Could you check a few things on this model? Use its own coordinates, in mm. Face numbers are marked on the shaded views. A direction names the side the tool comes from. Give positions to 0.01 mm unless a question says otherwise; leave off trailing zeros. Loops run counter-clockwise (first coordinate to the right, second up) from the corner with the lowest first, then second, coordinate; pieces in that order, holes last. Notation, with made-up numbers: (40, 22) - (84, 22) arc R22 cw to (84, 51) - close; hole circle Ø10 at (-3.5, -26.5). An arc over 180 degrees is marked (long way). One line per item, written item: value. Start each with the question number.
Q1. If I drill on line 1 (Y direction, x = -58, z = -8.25); line 2 (X direction, y = -24, z = -9.5); line 3 (X direction, y = 20.5, z = 1.25), over which ranges is the centre line in solid material (lowest first)? Write a range as from..to.
Q2. I'm going to push flat-ended pins straight in: P1, Ø13, axis at x = 17, y = -5, coming from the -Z side; P2, Ø2, axis at x = 47.5, y = 25, coming from the +Z side. Where does each tip first touch, or does it pass through?
Q3. I want a section at C-C (x = -19). Please give me the cut outline in (y, z).
Q4. I want a section at A-A (x = 0). Please give me the cut outline in (y, z), then the cut area to 3 significant figures.
Q5. I want a section at B-B (z = -1.75). Please give me the cut outline in (x, y), then the cut area to 3 significant figures.
Q6. For the marked faces 1, 2 and 3, which set-ups out of +Z, -Z, +X, -X, +Y, -Y let a thin tool reach every point of the face, with its end or its side?
Q7. If we mould it in two halves opening along Y, with no side actions, what happens to the marked faces 4, 5 and 6? For each: released by +Y, released by -Y, zero draft, split by the parting line, or undercut.
```python
from build123d import *

# Parameters (mm, degrees)
F0_W     = 126
F0_H     = 66
F0_W_2   = 120
F0_H_2   = 60
F1_DEPTH = 21
F2_W     = 126
F2_H     = 66
F3_DEPTH = 1
F0_R     = 12
F4_DEPTH = 8
F6_DEPTH = 22


with BuildPart() as f1:
    # F0 (on Top) → F1 (new body)
    with BuildSketch(Plane.XY):
        with Locations((-1.5, -1.5)):
            Rectangle(F0_W, F0_H)
        with Locations((-1.5, -1.5)):
            Rectangle(F0_W_2, F0_H_2, mode=Mode.SUBTRACT)
    extrude(amount=-F1_DEPTH)

    # F2 (on face) → F3 (join)
    with BuildSketch(Plane.XY):
        with Locations((-1.5, -1.5)):
            Rectangle(F2_W, F2_H)
    extrude(amount=F3_DEPTH)

    # F0 (on Top) → F4 (join)
    with BuildSketch(Plane.XY):
        with Locations((-40.3844975889, 14.0422494113)):
            Circle(F0_R)
        with Locations((0, 14)):
            Circle(F0_R)
        with Locations((-40.3844975889, -15.6422494113)):
            Circle(F0_R)
        with Locations((0, -15.6)):
            Circle(F0_R)
        with Locations((40.3844975889, -15.6422494113)):
            Circle(F0_R)
        with Locations((40.3844975889, 14.0422494113)):
            Circle(F0_R)
    extrude(amount=F4_DEPTH)

    # F5 (on face) → F6 (join)
    with BuildSketch(Plane.XY):
        with BuildLine():
            ThreePointArc((31.4784805761, 5.99968384), (32.8922690999, 2.7143222033), (33.3752768321, -0.8295602165))
            ThreePointArc((33.3752768321, -0.8295602165), (32.9180007232, -4.2794585958), (31.5777529034, -7.4910993057))
            ThreePointArc((31.5777529034, -7.4910993057), (33.0771463209, -6.123708691), (34.7855065256, -5.0285177832))
            ThreePointArc((34.7855065256, -5.0285177832), (35.2271141548, -2.9496471052), (35.3752768321, -0.8295602165))
            ThreePointArc((35.3752768321, -0.8295602165), (35.2220188743, 1.3264920966), (34.7653269231, 3.4391875409))
            ThreePointArc((34.7653269231, 3.4391875409), (33.0099261031, 4.57569273), (31.4784805761, 5.99968384))
        make_face()
        with BuildLine():
            ThreePointArc((30.044931449, 7.9518165828), (30.8064288175, 7.0085924135), (31.4784805761, 5.99968384))
            ThreePointArc((31.4784805761, 5.99968384), (33.0099261031, 4.57569273), (34.7653269231, 3.4391875409))
            ThreePointArc((34.7653269231, 3.4391875409), (32.4184567267, 8.1923854782), (28.5856333111, 11.8543733283))
            ThreePointArc((28.5856333111, 11.8543733283), (29.1446126861, 9.8392757768), (30.044931449, 7.9518165828))
        make_face()
        with BuildLine():
            ThreePointArc((34.7855065256, -5.0285177832), (33.0771463209, -6.123708691), (31.5777529034, -7.4910993057))
            ThreePointArc((31.5777529034, -7.4910993057), (30.8212956484, -8.6474276201), (29.948463719, -9.718635897))
            ThreePointArc((29.948463719, -9.718635897), (29.0995516946, -11.5618087289), (28.5733528944, -13.5216690648))
            ThreePointArc((28.5733528944, -13.5216690648), (32.4355688891, -9.8281570151), (34.7855065256, -5.0285177832))
        make_face()
        with BuildLine():
            ThreePointArc((10.5845976874, 8.3461259481), (20.4011056558, 12.410159384), (30.044931449, 7.9518165828))
            ThreePointArc((30.044931449, 7.9518165828), (29.1446126861, 9.8392757768), (28.5856333111, 11.8543733283))
            ThreePointArc((28.5856333111, 11.8543733283), (20.2186418923, 14.4126354365), (11.8233794228, 11.9487323369))
            ThreePointArc((11.8233794228, 11.9487323369), (11.3478655588, 10.0979560153), (10.5845976874, 8.3461259481))
        make_face()
        with BuildLine():
            ThreePointArc((28.5733528944, -13.5216690648), (29.0995516946, -11.5618087289), (29.948463719, -9.718635897))
            ThreePointArc((29.948463719, -9.718635897), (20.3778358891, -14.0697308571), (10.652789482, -10.0756831869))
            ThreePointArc((10.652789482, -10.0756831869), (11.3821848264, -11.7992278973), (11.8347224415, -13.615221742))
            ThreePointArc((11.8347224415, -13.615221742), (20.2180287599, -16.0717593087), (28.5733528944, -13.5216690648))
        make_face()
        with BuildLine():
            ThreePointArc((8.5383868776, 5.5681585921), (9.4706325231, 7.0240682624), (10.5845976874, 8.3461259481))
            ThreePointArc((10.5845976874, 8.3461259481), (11.3478655588, 10.0979560153), (11.8233794228, 11.9487323369))
            ThreePointArc((11.8233794228, 11.9487323369), (7.86032363, 8.2101986383), (5.4651898622, 3.3167561214))
            ThreePointArc((5.4651898622, 3.3167561214), (7.0917024506, 4.3197233329), (8.5383868776, 5.5681585921))
        make_face()
        with BuildLine():
            ThreePointArc((11.8347224415, -13.615221742), (11.3821848264, -11.7992278973), (10.652789482, -10.0756831869))
            ThreePointArc((10.652789482, -10.0756831869), (9.455680238, -8.6628486697), (8.46736073, -7.0968357497))
            ThreePointArc((8.46736073, -7.0968357497), (7.0422594659, -5.8836950637), (5.4458638506, -4.9068916156))
            ThreePointArc((5.4458638506, -4.9068916156), (7.8431131072, -9.8459070996), (11.8347224415, -13.615221742))
        make_face()
        with BuildLine():
            ThreePointArc((8.46736073, -7.0968357497), (6.8906107626, -0.7552968983), (8.5383868776, 5.5681585921))
            ThreePointArc((8.5383868776, 5.5681585921), (7.0917024506, 4.3197233329), (5.4651898622, 3.3167561214))
            ThreePointArc((5.4651898622, 3.3167561214), (4.8904446173, -0.7937397736), (5.4458638506, -4.9068916156))
            ThreePointArc((5.4458638506, -4.9068916156), (7.0422594659, -5.8836950637), (8.46736073, -7.0968357497))
        make_face()
        with BuildLine():
            ThreePointArc((-8.5383868776, 5.5681585921), (-7.0917024506, 4.3197233329), (-5.4651898622, 3.3167561214))
            ThreePointArc((-5.4651898622, 3.3167561214), (-7.86032363, 8.2101986383), (-11.8233794228, 11.9487323369))
            ThreePointArc((-11.8233794228, 11.9487323369), (-11.3478655588, 10.0979560153), (-10.5845976874, 8.3461259481))
            ThreePointArc((-10.5845976874, 8.3461259481), (-9.4706325231, 7.0240682624), (-8.5383868776, 5.5681585921))
        make_face()
        with BuildLine():
            ThreePointArc((-4.8904025274, -0.8295602165), (-5.034783168, 1.2634232792), (-5.4651898622, 3.3167561214))
            ThreePointArc((-5.4651898622, 3.3167561214), (-7.0917024506, 4.3197233329), (-8.5383868776, 5.5681585921))
            ThreePointArc((-8.5383868776, 5.5681585921), (-7.3090150887, 2.4737206667), (-6.8904025274, -0.8295602165))
            ThreePointArc((-6.8904025274, -0.8295602165), (-7.2906920093, -4.0608734086), (-8.46736073, -7.0968357497))
            ThreePointArc((-8.46736073, -7.0968357497), (-7.0422594659, -5.8836950637), (-5.4458638506, -4.9068916156))
            ThreePointArc((-5.4458638506, -4.9068916156), (-5.0299062498, -2.8870567912), (-4.8904025274, -0.8295602165))
        make_face()
        with BuildLine():
            ThreePointArc((-10.5845976874, 8.3461259481), (-11.3478655588, 10.0979560153), (-11.8233794228, 11.9487323369))
            ThreePointArc((-11.8233794228, 11.9487323369), (-20.2186418923, 14.4126354365), (-28.5856333111, 11.8543733283))
            ThreePointArc((-28.5856333111, 11.8543733283), (-29.1446126861, 9.8392757768), (-30.044931449, 7.9518165828))
            ThreePointArc((-30.044931449, 7.9518165828), (-20.4011056558, 12.410159384), (-10.5845976874, 8.3461259481))
        make_face()
        with BuildLine():
            ThreePointArc((-11.8347224415, -13.615221742), (-7.8431131072, -9.8459070996), (-5.4458638506, -4.9068916156))
            ThreePointArc((-5.4458638506, -4.9068916156), (-7.0422594659, -5.8836950637), (-8.46736073, -7.0968357497))
            ThreePointArc((-8.46736073, -7.0968357497), (-9.455680238, -8.6628486697), (-10.652789482, -10.0756831869))
            ThreePointArc((-10.652789482, -10.0756831869), (-11.3821848264, -11.7992278973), (-11.8347224415, -13.615221742))
        make_face()
        with BuildLine():
            ThreePointArc((-28.5733528944, -13.5216690648), (-20.2180287599, -16.0717593087), (-11.8347224415, -13.615221742))
            ThreePointArc((-11.8347224415, -13.615221742), (-11.3821848264, -11.7992278973), (-10.652789482, -10.0756831869))
            ThreePointArc((-10.652789482, -10.0756831869), (-20.3778358891, -14.0697308571), (-29.948463719, -9.718635897))
            ThreePointArc((-29.948463719, -9.718635897), (-29.0995516946, -11.5618087289), (-28.5733528944, -13.5216690648))
        make_face()
        with BuildLine():
            ThreePointArc((-30.044931449, 7.9518165828), (-29.1446126861, 9.8392757768), (-28.5856333111, 11.8543733283))
            ThreePointArc((-28.5856333111, 11.8543733283), (-32.4184567267, 8.1923854782), (-34.7653269231, 3.4391875409))
            ThreePointArc((-34.7653269231, 3.4391875409), (-33.0099261031, 4.57569273), (-31.4784805761, 5.99968384))
            ThreePointArc((-31.4784805761, 5.99968384), (-30.8064288175, 7.0085924135), (-30.044931449, 7.9518165828))
        make_face()
        with BuildLine():
            ThreePointArc((-34.7855065256, -5.0285177832), (-32.4355688891, -9.8281570151), (-28.5733528944, -13.5216690648))
            ThreePointArc((-28.5733528944, -13.5216690648), (-29.0995516946, -11.5618087289), (-29.948463719, -9.718635897))
            ThreePointArc((-29.948463719, -9.718635897), (-30.8212956484, -8.6474276201), (-31.5777529034, -7.4910993057))
            ThreePointArc((-31.5777529034, -7.4910993057), (-33.0771463209, -6.123708691), (-34.7855065256, -5.0285177832))
        make_face()
        with BuildLine():
            ThreePointArc((-31.4784805761, 5.99968384), (-33.0099261031, 4.57569273), (-34.7653269231, 3.4391875409))
            ThreePointArc((-34.7653269231, 3.4391875409), (-35.3752335492, -0.7932356825), (-34.7855065256, -5.0285177832))
            ThreePointArc((-34.7855065256, -5.0285177832), (-33.0771463209, -6.123708691), (-31.5777529034, -7.4910993057))
            ThreePointArc((-31.5777529034, -7.4910993057), (-33.3749183212, -0.7321179887), (-31.4784805761, 5.99968384))
        make_face()
    extrude(amount=-F6_DEPTH)


solid = f1.part
```
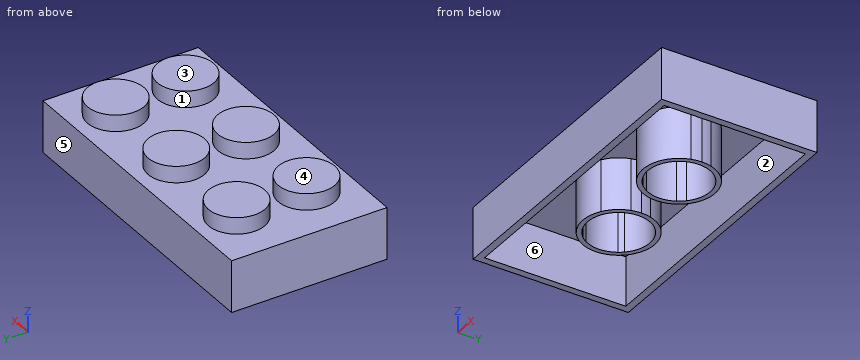
Worked answers:
1. line 1: y = -34.5..-31.5, 28.5..31.5
1. line 2: x = -64.5..-61.5, 58.5..61.5
1. line 3: x = -50.5..-30.27, -10.09..10.09, 30.27..50.5
2. P1: stops at z = 0
2. P2: stops at z = 1
3. outline: (-34.5, -21) - (-31.5, -21) - (-31.5, 0) - (-16.03, 0) - (-16.03, -22) - (-14.02, -22) - (-14.02, 0) - (12.36, 0) - (12.36, -22) - (14.37, -22) - (14.37, 0) - (28.5, 0) - (28.5, -21) - (31.5, -21) - (31.5, 1) - (-34.5, 1) - close
4. outline: (-34.5, -21) - (-31.5, -21) - (-31.5, 0) - (28.5, 0) - (28.5, -21) - (31.5, -21) - (31.5, 1) - (26, 1) - (26, 8) - (2, 8) - (2, 1) - (-3.6, 1) - (-3.6, 8) - (-27.6, 8) - (-27.6, 1) - (-34.5, 1) - close
4. area: 528 mm²
5. outline: (-64.5, -34.5) - (61.5, -34.5) - (61.5, 31.5) - (-64.5, 31.5) - close; circle Ø30.48 at (-20.13, -0.83); circle Ø30.48 at (20.13, -0.83); hole (-61.5, -31.5) - (58.5, -31.5) - (58.5, 28.5) - (-61.5, 28.5) - close; hole circle Ø26.48 at (-20.13, -0.83); hole circle Ø26.48 at (20.13, -0.83)
5. area: 1,470 mm²
6. face 1: +Z
6. face 2: -Z
6. face 3: +Z, +X, -X, +Y, -Y
7. face 4: zero draft
7. face 5: released by +Y
7. face 6: undercut
